Read the model definition and answer for the solid it produces. Units are mm, in the model's axes. A direction names the side the tool comes from. Round coordinates to 2 decimals unless told otherwise and drop trailing zeros. Loops run counter-clockwise (first coordinate to the right, second up) from the corner with the lowest first, then second, coordinate; pieces in that order, holes last. Notation, with made-up numbers: (-30, 63) - (10, 63) arc R11 ccw to (10, 79) - close; hole circle Ø5 at (79.5, 36.25). An arc over 180 degrees is marked (long way). Use CSV: the item, a comma, the result in double quotes. Start each with the question number.
1. Determine the mould class of faces 1 (the flat face through (25, 3, 0)), 2 (the flat face through (0, 3, -25)), 3 (the flat face through (8.266, 14.605, -4.684)) for opening direction Z: +Z half, -Z half, draft (parallel to the pull), parting line (faces both ways), or undercut.
2. A tool of negligible diameter and unlimited length cuts with its end or side. For faces 4 (the flat face through (18, 5, 14)), 5 (the flat face through (0, 14, 22)), 6 (the flat face through (0, 15, 9.5)), from which of +Z, -Z, +X, -X, +Y, -Y can it reach the whole face along a straight path? Write none if from no direction.
3. Find section D-D (x = -14). Give the vertices of the cut face in (y, z), and give its area (3 significant figures).
4. Find section A-A (x = 0). Give the vertices of the cut face in (y, z).
5. Find section B-B (y = 12). Give the vertices of the cut face in (x, z), and give its area (3 significant figures).
6. Consider line 1 along Z through (x, y) = (14, 3.65); line 2 along Z through (x, y) = (14, 9.5); line 3 along Z through (x, y) = (4.5, 9). Determine where each line is inside the solid, lowest interval first.
7. Given pin 1 Ø3.5 at (x, y) = (0.5, 13) entering from -Z; pin 2 Ø1.5 at (y, z) = (18, 14) entering from +X; pin 3 Ø4.5 at (y, z) = (14.5, -6) entering from -X, each flat-ended and moving along its own axis, determine where each tip first touches the part or whether it passes through.
8. Find section C-C (z = 14). Give the vertices of the cut face in (x, y).
from build123d import *

# Parameters (mm, degrees)
F0_W      = 50
F0_H      = 50
F1_DEPTH  = 7
F2_W      = 44
F2_H      = 44
F3_DEPTH  = 15
F4_R      = 3
F5_DEPTH  = 25
F7_R      = 7
F8_DEPTH  = 25
F9_R      = 7
F10_DEPTH = 15
F6_R      = 8.5
F11_DEPTH = 5


# Not quite as in the source:
# - a feature names something its author has since deleted; it is built from what else it names


with BuildPart() as f1:
    # F0 (on Front) → F1 (new body)
    with BuildSketch(Plane.XZ):
        Rectangle(F0_W, F0_H)
    extrude(amount=-F1_DEPTH)

    # F2 (on face) → F3 (join)
    with BuildSketch(Plane(origin=(0, 7, 0), x_dir=(-1, 0, 0), z_dir=(0, 1, 0))):
        Rectangle(F2_W, F2_H)
    extrude(amount=F3_DEPTH)

    # F4 (on face) → F5 (cut)
    with BuildSketch(Plane(origin=(0, 22, 0), x_dir=(-1, 0, 0), z_dir=(0, 1, 0))):
        with Locations((-14, 14)):
            Circle(F4_R)
        with Locations((14, 14)):
            Circle(F4_R)
        with Locations((14, -14)):
            Circle(F4_R)
        with Locations((-14, -14)):
            Circle(F4_R)
    extrude(amount=-F5_DEPTH, mode=Mode.SUBTRACT)

    # F7 (on face) → F8 (cut)
    with BuildSketch(Plane.XZ):
        Circle(F7_R)
    extrude(amount=-F8_DEPTH, mode=Mode.SUBTRACT)

    # F9 (on face) → F10 (cut)
    with BuildSketch(Plane(origin=(0, 22, 0), x_dir=(-1, 0, 0), z_dir=(0, 1, 0))):
        Polygon((-5.4848275573, -9.5), (5.4848275573, -9.5), (10.9696551146, 0), (5.4848275573, 9.5), (-5.4848275573, 9.5), (-10.9696551146, 0), align=None)
        Circle(F9_R, mode=Mode.SUBTRACT)
    extrude(amount=-F10_DEPTH, mode=Mode.SUBTRACT)

    # F6 (on face) → F11 (cut)
    with BuildSketch(Plane.XZ):
        with Locations((-14, 14)):
            Circle(F6_R)
        with Locations((-14, -14)):
            Circle(F6_R)
        with Locations((14, -14)):
            Circle(F6_R)
        with Locations((14, 14)):
            Circle(F6_R)
    extrude(amount=-F11_DEPTH, mode=Mode.SUBTRACT)


solid = f1.part
Filled sheet:
1,face 1,"draft"
1,face 2,"-Z half"
1,face 3,"undercut"
2,face 4,"-Y"
2,face 5,"+Z, +X, -X, +Y"
2,face 6,"+Y"
3,outline,"(0, -25) - (7, -25) - (7, -22) - (22, -22) - (22, -17) - (5, -17) - (5, -22.5) - (0, -22.5) - close; (0, -5.5) - (5, -5.5) - (5, -11) - (22, -11) - (22, 11) - (5, 11) - (5, 5.5) - (0, 5.5) - close; (0, 22.5) - (5, 22.5) - (5, 17) - (22, 17) - (22, 22) - (7, 22) - (7, 25) - (0, 25) - close"
3,area,"636 mm²"
4,outline,"(0, -25) - (7, -25) - (7, -22) - (22, -22) - (22, -9.5) - (7, -9.5) - (7, -7) - (0, -7) - close; (0, 7) - (7, 7) - (7, 9.5) - (22, 9.5) - (22, 22) - (7, 22) - (7, 25) - (0, 25) - close"
5,outline,"(-22, -22) - (22, -22) - (22, 22) - (-22, 22) - close; hole circle Ø6 at (-14, -14); hole circle Ø6 at (-14, 14); hole (-10.97, 0) - (-5.48, -9.5) - (5.48, -9.5) - (10.97, 0) - (5.48, 9.5) - (-5.48, 9.5) - close; hole circle Ø6 at (14, -14); hole circle Ø6 at (14, 14)"
5,area,"1,510 mm²"
6,line 1,"z = -25 to -22.5, -5.5 to 5.5, 22.5 to 25"
6,line 2,"z = -22 to -17, -11 to 11, 17 to 22"
6,line 3,"z = -22 to -9.5, 9.5 to 22"
7,pin 1,"stops at z = -22"
7,pin 2,"stops at x = 22"
7,pin 3,"stops at x = -22"
8,outline,"(-25, 0) - (-22.5, 0) - (-22.5, 5) - (-17, 5) - (-17, 22) - (-22, 22) - (-22, 7) - (-25, 7) - close; (-11, 5) - (-5.5, 5) - (-5.5, 0) - (5.5, 0) - (5.5, 5) - (11, 5) - (11, 22) - (-11, 22) - close; (17, 5) - (22.5, 5) - (22.5, 0) - (25, 0) - (25, 7) - (22, 7) - (22, 22) - (17, 22) - close"
